```python
from build123d import *

# Parameters (mm, degrees)
BOSS_EXTRUDE1_DEPTH = 19.05
CUT_EXTRUDE1_DEPTH  = 9.525
CUT_EXTRUDE2_DEPTH  = 9.525
FILLET2_R           = 6.35
SKETCH5_R           = 4.7625
CUT_EXTRUDE3_DEPTH  = 3.175
SKETCH6_W           = 25.908
SKETCH6_H           = 10.922
CUT_EXTRUDE4_DEPTH  = 2.032


with BuildPart() as part:
    # Sketch1 → Boss-Extrude1 (new body)
    with BuildSketch(Plane(origin=(0, 0, 0), x_dir=(1, 0, 0), z_dir=(0, 1, 0))):
        Polygon((-101.6, -19.05), (-76.2, -44.45), (76.2, -44.45), (101.6, -19.05), (101.6, 19.05), (76.2, 44.45), (-76.2, 44.45), (-101.6, 19.05), align=None)
    extrude(amount=BOSS_EXTRUDE1_DEPTH)

    # Sketch2 → Cut-Extrude1 (cut)
    with BuildSketch(Plane(origin=(0, 19.05, 0), x_dir=(1, 0, 0), z_dir=(0, 1, 0))):
        with BuildLine():
            Line((-76.2, 27.305), (82.55, 27.305))
            ThreePointArc((82.55, 27.305), (87.63, 22.225), (82.55, 17.145))
            Line((82.55, 17.145), (-76.2, 17.145))
            ThreePointArc((-76.2, 17.145), (-81.28, 22.225), (-76.2, 27.305))
        make_face()
        with BuildLine():
            Line((92.075, -5.08), (-66.675, -5.08))
            ThreePointArc((-66.675, -5.08), (-71.755, 0), (-66.675, 5.08))
            Line((-66.675, 5.08), (92.075, 5.08))
            ThreePointArc((92.075, 5.08), (97.155, 0), (92.075, -5.08))
        make_face()
        with BuildLine():
            Line((-76.2, -17.145), (82.55, -17.145))
            ThreePointArc((82.55, -17.145), (87.63, -22.225), (82.55, -27.305))
            Line((82.55, -27.305), (-76.2, -27.305))
            ThreePointArc((-76.2, -27.305), (-81.28, -22.225), (-76.2, -17.145))
        make_face()
    extrude(amount=-CUT_EXTRUDE1_DEPTH, mode=Mode.SUBTRACT)

    # Sketch3 → Cut-Extrude2 (cut)
    with BuildSketch(Plane(origin=(0, 19.05, 0), x_dir=(1, 0, 0), z_dir=(0, 1, 0))):
        Polygon((-87.88238686, 31.75), (-79.375, 0), (-87.88238686, -31.75), (-49.78238686, -31.75), (-41.275, 0), (-49.78238686, 31.75), align=None)
    extrude(amount=-CUT_EXTRUDE2_DEPTH, mode=Mode.SUBTRACT)

    # Fillet2
    # the kernel refuses this fillet: 6.35 mm, written as the material it adds along each edge
    with BuildSketch(Plane(origin=(-49.78238686, 19.05, 31.75), x_dir=(-1, 0, 0), z_dir=(0, -1, 0))) as fillet2_piece_1:
        with BuildLine():
            CenterArc((4.866479769, 6.35), FILLET2_R, 197.457603124, 72.542396876)
            Line((-1.19103416, 4.445), (0, 0))
            Line((0, 0), (4.866479769, 0))
        make_face()
    extrude(amount=9.525)
    with BuildSketch(Plane(origin=(-49.78238686, 19.05, -31.75), x_dir=(0.2588190451025257, 0, 0.9659258262890671), z_dir=(0, -1, 0))) as fillet2_piece_2:
        with BuildLine():
            CenterArc((4.87409135, 6.344159428), FILLET2_R, 195, 72.542396876)
            Line((-1.259537647, 4.700658492), (0, 0))
            Line((0, 0), (4.601802622, 0))
        make_face()
    extrude(amount=9.525)
    with BuildSketch(Plane(origin=(-87.88238686, 19.05, 31.75), x_dir=(0.2588190451025169, 0, -0.9659258262890692), z_dir=(0, -1, 0)), Plane(origin=(-87.88238686, 19.05, -31.75), x_dir=(1, 0, 0), z_dir=(0, -1, 0))) as fillet2_piece_3:
        with BuildLine():
            CenterArc((FILLET2_R * 1.30322537284, FILLET2_R), FILLET2_R, 165, 105)
            Line((FILLET2_R * 0.337299546552, FILLET2_R * 1.2588190451), (0, 0))
            Line((0, 0), (FILLET2_R * 1.30322537284, 0))
        make_face()
    extrude(amount=9.525)

    # Sketch5 → Cut-Extrude3 (cut)
    with BuildSketch(Plane(origin=(0, 19.05, 0), x_dir=(1, 0, 0), z_dir=(0, 1, 0))):
        with Locations(Location((-63.5, -38.735, 0), (0, 0, 270))):
            Circle(SKETCH5_R)
        with Locations(Location((63.5, -38.735, 0), (0, 0, 270))):
            Circle(SKETCH5_R)
    extrude(amount=-CUT_EXTRUDE3_DEPTH, mode=Mode.SUBTRACT)

    # Sketch6 → Cut-Extrude4 (cut)
    with BuildSketch(Plane(origin=(0, 19.05, 0), x_dir=(1, 0, 0), z_dir=(0, 1, 0))):
        with Locations((-50.8, 38.989)):
            Rectangle(SKETCH6_W, SKETCH6_H)
    cut_extrude4 = extrude(amount=-CUT_EXTRUDE4_DEPTH, mode=Mode.SUBTRACT)

    # Mirror1: Cut-Extrude4 across plane
    add(cut_extrude4.mirror(Plane(origin=(0, 0, 0), x_dir=(0, 0, 1), z_dir=(1, 0, 0))), mode=Mode.SUBTRACT)


solid = part.part
```
Design review of the part built by this model. Coordinates are the model's own, in mm. A direction names the side the tool comes from. Round coordinates to 2 decimals unless told otherwise and drop trailing zeros. Write each loop counter-clockwise with the first axis right and the second up, starting at its lowest first coordinate (ties: lowest second). Pieces come first, ordered by that corner, then holes.
Item 1: Clearance check with flat-ended pins moving along their axes: pin 1 Ø2 at (y, z) = (12, -26) entering from -X; pin 2 Ø0.6 at (x, y) = (-57, 18) entering from -Z; pin 3 Ø1.6 at (y, z) = (18.5, -39) entering from +X. State where each tip first meets the part, or that it passes through.
Item 2: For faces 4 (the flat face through (5, 19.05, -14)), 5 (the flat face through (18, 14, 27.305)), list the 3-axis set-ups (+Z, -Z, +X, -X, +Y, -Y) from which the entire face can be reached by the end or side of a thin tool; tool diameter is ignored.
Item 3: We need section B-B on x = -22. Write out the cut boundary in (y, z) (3 decimals).
Item 4: The part is to be moulded in two halves that separate along Z. For faces 1 (the flat face through (-82.6, 14.35, -12.04)), 2 (the flat face through (-101.6, 9, 0)), 3 (the flat face through (1, 9, -44.45)), say which applies: +Z half, -Z half, draft (parallel to the pull), parting line (faces both ways), or undercut.
Item 5: We need section C-C on z = 12. Write out the cut boundary in (x, y) (3 decimals).
Item 6: For probe 1 along Z at (x, y) = (57.5, 13.25) (3 decimals); probe 2 along X at (y, z) = (9.75, 11.5); probe 3 along X at (y, z) = (11.5, -25.5), list the stretches that pass through material, from the lowest coordinate up.
Item 7: We need section A-A on y = 5.25. Write out the cut boundary in (x, z), and give its area (3 significant figures).
Returned:
1. pin 1: stops at x = -95.65
1. pin 2: stops at z = -33.53
1. pin 3: stops at x = 82.45
2. face 4: +Z, -Z, +X, -X, +Y
2. face 5: +Y
3. outline: (0, -44.45) - (19.05, -44.45) - (19.05, -27.305) - (9.525, -27.305) - (9.525, -17.145) - (19.05, -17.145) - (19.05, -5.08) - (9.525, -5.08) - (9.525, 5.08) - (19.05, 5.08) - (19.05, 17.145) - (9.525, 17.145) - (9.525, 27.305) - (19.05, 27.305) - (19.05, 44.45) - (0, 44.45) - close
4. face 1: undercut
4. face 2: draft
4. face 3: -Z half
5. outline: (-101.6, 0) - (101.6, 0) - (101.6, 19.05) - (-44.49, 19.05) - (-44.49, 9.525) - (-82.59, 9.525) - (-82.59, 19.05) - (-101.6, 19.05) - close
6. probe 1: z = -44.45 to -27.305, -17.145 to -5.08, 5.08 to 17.145, 27.305 to 44.45
6. probe 2: x = -101.6 to -82.46, -44.36 to 101.6
6. probe 3: x = -95.15 to -85.96, 86.43 to 95.15
7. outline: (-101.6, -19.05) - (-76.2, -44.45) - (76.2, -44.45) - (101.6, -19.05) - (101.6, 19.05) - (76.2, 44.45) - (-76.2, 44.45) - (-101.6, 19.05) - close
7. area: 16,800 mm2
